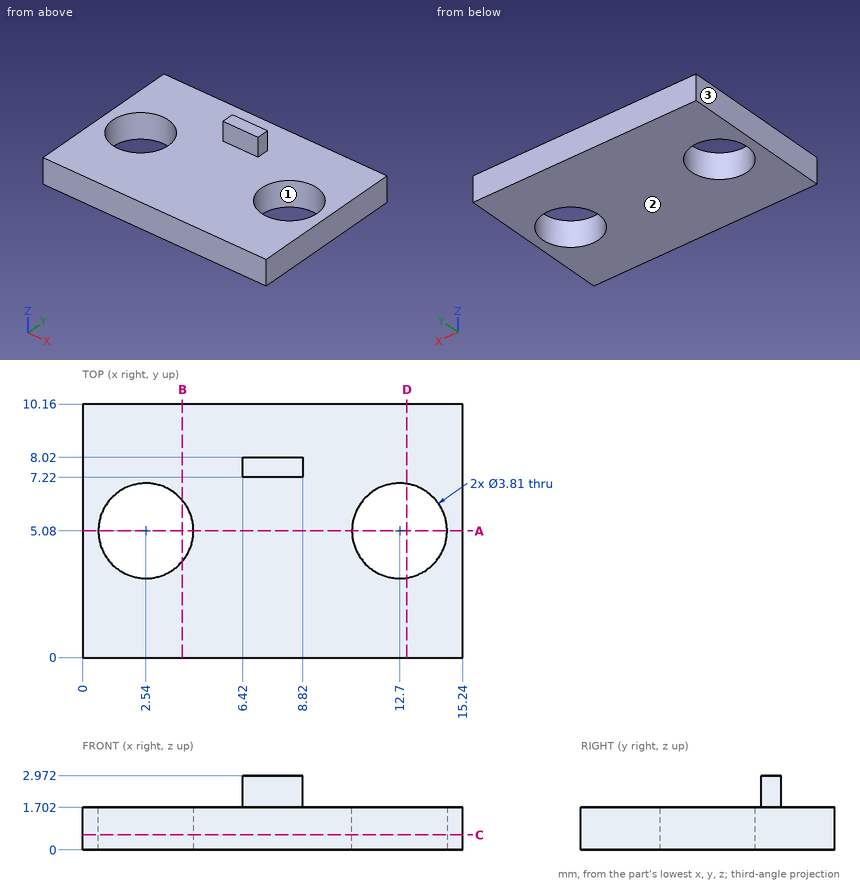
Source: three-view drawing plus pictorial views. Frame: mm from the lowest corner of the part. Round coordinates to 2 decimals unless told otherwise and drop trailing zeros. Loops run counter-clockwise (first coordinate to the right, second up) from the corner with the lowest first, then second, coordinate; pieces in that order, holes last. Notation, with made-up numbers: (13.5, 48.5) - (71.5, 48.5) arc R29 cw to (71.5, 70.5) - close; hole circle Ø9 at (-32, 29). An arc over 180 degrees is marked (long way). Write each question's results on one line, items separated by ' | '. Start each with the question number.
1) Cut plane C-C on z = 0.6. Return loops of the section in (x, y) (3 decimals).
2) Cut plane B-B on x = 4. Return loops of the section in (y, z).
3) Cut plane A-A on y = 5.08. Return loops of the section in (x, z) (1 decimal), then the cut area to 3 significant figures.
4) Cut plane D-D on x = 13. Return loops of the section in (y, z), then the cut area to 3 significant figures.
5) First-contact query: P1, Ø1.5, axis at x = 8, z = 2.5, coming from the +Y side; P2, Ø5, axis at x = 6, y = 2.5, coming from the +Z side; P3, Ø1.4, axis at x = 7, z = 2.5, coming from the -Y side. Flat tips, straight axial feed; report the tip coordinate or a pass-through.
6) Line query: probe 1 along Y at (x, z) = (12.7, 0.65) (3 decimals); probe 2 along Z at (x, y) = (3.75, 9); probe 3 along X at (y, z) = (5.5, 0.35). Output: solid intervals per line, ascending. Write a range as [from, to].
7) Mould query, pull axis X, two halves, no side actions, for the marked faces 1, 2 and 3. Classes: released by +X, released by -X, zero draft, split by the parting line, or undercut.
Verdict:
1) outline: (0, 0) - (15.24, 0) - (15.24, 10.16) - (0, 10.16) - close; hole circle Ø3.81 at (2.54, 5.08); hole circle Ø3.81 at (12.7, 5.08)
2) outline: (0, 0) - (3.86, 0) - (3.86, 1.7) - (0, 1.7) - close; (6.3, 0) - (10.16, 0) - (10.16, 1.7) - (6.3, 1.7) - close
3) outline: (0, 0) - (0.6, 0) - (0.6, 1.7) - (0, 1.7) - close; (4.4, 0) - (10.8, 0) - (10.8, 1.7) - (4.4, 1.7) - close; (14.6, 0) - (15.2, 0) - (15.2, 1.7) - (14.6, 1.7) - close | area: 13.0 mm2
4) outline: (0, 0) - (3.2, 0) - (3.2, 1.7) - (0, 1.7) - close; (6.96, 0) - (10.16, 0) - (10.16, 1.7) - (6.96, 1.7) - close | area: 10.9 mm2
5) P1: stops at y = 8.02 | P2: stops at z = 1.7 | P3: stops at y = 7.22
6) probe 1: y = [0, 3.175], [6.985, 10.16] | probe 2: z = [0, 1.7] | probe 3: x = [0, 0.68], [4.4, 10.84], [14.56, 15.24]
7) face 1: undercut | face 2: zero draft | face 3: released by -X
